Here's the drawing with two shaded views (mm, measured from the low corner). I have some questions. A direction names the side the tool comes from. Coordinates: 2 decimals unless noted, no trailing zeros. Order: outer loops, then holes, each group sorted by start corner. A loop starts at its lowest first (then second) coordinate and runs counter-clockwise, first axis right, second up. Notation, with made-up numbers: (36.5, -37.5) -> (57.5, -37.5) arc R13 ccw to (57.5, -31.5) -> close; hole circle Ø7 at (71, 68). An arc over 180 degrees is marked (long way). One line per item, written item: value. Start each with the question number.
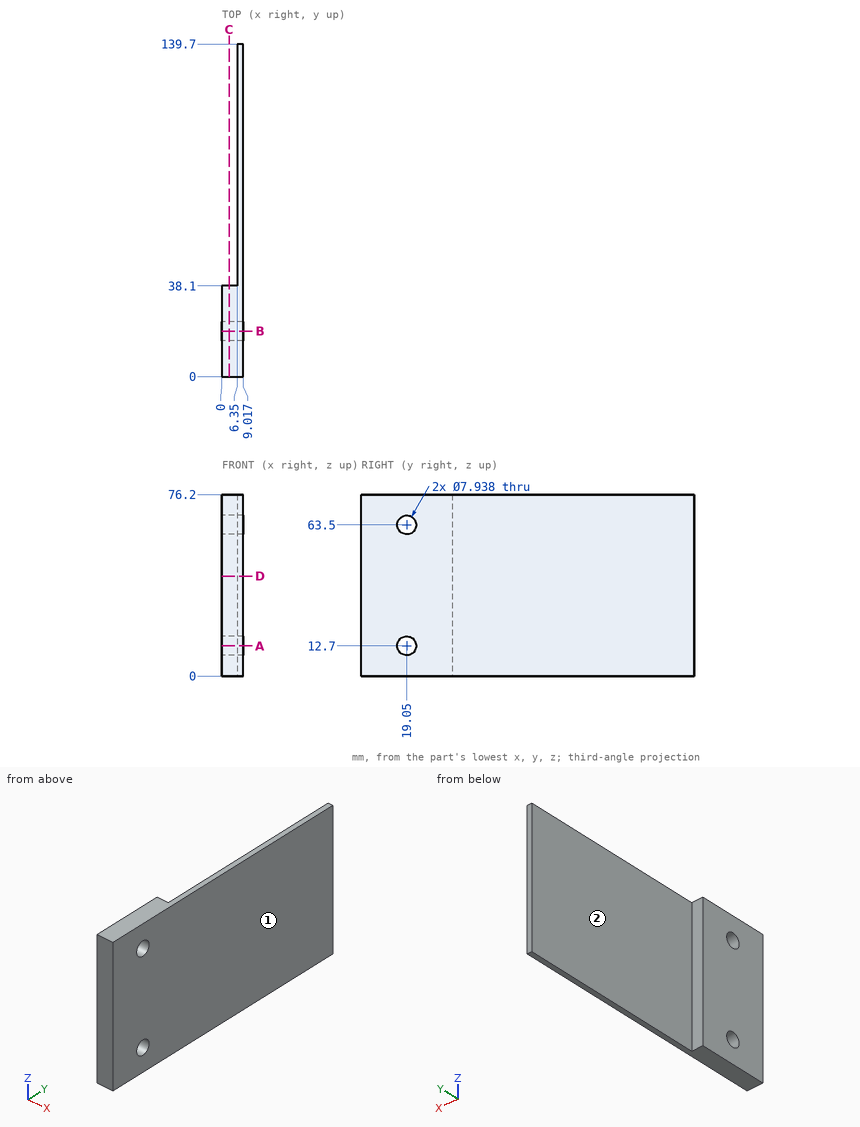
Q1. Imagine slicing it at C-C (x = 3). Write out the boundary of the cut face in (y, z), plus the area to 3 significant figures.
Q2. Imagine slicing it at D-D (z = 42). Write out the boundary of the cut face in (x, y).
Q3. Imagine slicing it at B-B (y = 19.05). Write out the boundary of the cut face in (x, z).
Q4. Imagine slicing it at A-A (z = 12.7). Write out the boundary of the cut face in (x, y).
Q5. I need wall thicknesses on line 1 (Z direction, x = 5.75, y = 19.05); line 2 (Y direction, x = 7.5, z = 64); line 3 (Z direction, x = 1.25, y = 18). Which ranges of each line are inside material? Lowest first, please.
Q6. For P1, Ø1.5, axis at x = 2, z = 46, coming from the +Y side; P2, Ø2, axis at y = 116.5, z = 27, coming from the -X side, each with a flat end and sliding along its axis, tell me the tip position at first contact or that it passes through.
Q7. For the marked faces 1 and 2, which set-ups out of +Z, -Z, +X, -X, +Y, -Y let a thin tool reach every point of the face, with its end or its side?
Completed:
1. outline: (0, 0) -> (38.1, 0) -> (38.1, 76.2) -> (0, 76.2) -> close; hole circle Ø7.94 at (19.05, 12.7); hole circle Ø7.94 at (19.05, 63.5)
1. area: 2,800 mm2
2. outline: (0, 0) -> (9.02, 0) -> (9.02, 139.7) -> (6.35, 139.7) -> (6.35, 38.1) -> (0, 38.1) -> close
3. outline: (0, 0) -> (9.02, 0) -> (9.02, 8.73) -> (0, 8.73) -> close; (0, 16.67) -> (9.02, 16.67) -> (9.02, 59.53) -> (0, 59.53) -> close; (0, 67.47) -> (9.02, 67.47) -> (9.02, 76.2) -> (0, 76.2) -> close
4. outline: (0, 0) -> (9.02, 0) -> (9.02, 15.08) -> (0, 15.08) -> close; (0, 23.02) -> (9.02, 23.02) -> (9.02, 139.7) -> (6.35, 139.7) -> (6.35, 38.1) -> (0, 38.1) -> close
5. line 1: z = 0 to 8.73, 16.67 to 59.53, 67.47 to 76.2
5. line 2: y = 0 to 15.11, 22.99 to 139.7
5. line 3: z = 0 to 8.87, 16.53 to 59.67, 67.33 to 76.2
6. P1: stops at y = 38.1
6. P2: stops at x = 6.35
7. face 1: +Z, -Z, +X, +Y, -Y
7. face 2: +Z, -Z, -X, +Y
